The listing builds one solid part. Answer for the finished solid, in the listing's coordinates (mm). A direction names the side the tool comes from. Round coordinates to 2 decimals unless told otherwise and drop trailing zeros. Write each loop counter-clockwise with the first axis right and the second up, starting at its lowest first coordinate (ties: lowest second). Pieces come first, ordered by that corner, then holes.
from build123d import *

# Parameters (mm, degrees)
SKETCH1_W               = 10
SKETCH1_H               = 10
BOSS_EXTRUDE1_DEPTH     = 5
SKETCH4_R               = 3
CUT_EXTRUDE1_DEPTH      = 4
SKETCH5_R               = 4.05
BOSS_EXTRUDE2_DEPTH     = 30
CUT_EXTRUDE2_DEPTH      = 106.032848815
CUT_EXTRUDE2_DEPTH_BACK = 106.032848815
SKETCH6_W               = 26.365617629
SKETCH6_H               = 20
SKETCH8_W               = 10
SKETCH8_H               = 8.643528748
BOSS_EXTRUDE3_DEPTH     = 40
SKETCH9_R               = 2.5
BOSS_EXTRUDE4_DEPTH     = 10
CUT_EXTRUDE3_DEPTH      = 99.974452188
CUT_EXTRUDE3_DEPTH_BACK = 99.974452188
CUT_EXTRUDE5_DEPTH      = 99.974452188
CUT_EXTRUDE5_DEPTH_BACK = 99.974452188
SKETCH13_W              = 27.262735852
SKETCH13_H              = 14.70463532
SKETCH14_W              = 24
SKETCH14_H              = 18
BOSS_EXTRUDE5_DEPTH     = 10
SKETCH15_R              = 2.246907778
BOSS_EXTRUDE6_DEPTH     = 9
SKETCH16_W              = 26.867537366
SKETCH16_H              = 22.487326792
CUT_EXTRUDE6_DEPTH      = 5.25


with BuildPart() as part:
    # Sketch1 → Boss-Extrude1 (new, symmetric)
    with BuildSketch(Plane(origin=(0, 0, 0), x_dir=(0, 0, -1), z_dir=(1, 0, 0))):
        with BuildLine():
            Line((-40, -40), (-40, -50))
            Line((-40, -50), (-3.5, -50))
            ThreePointArc((-3.5, -50), (0, -46.5), (3.5, -50))
            Line((3.5, -50), (40, -50))
            Line((40, -50), (40, -40))
            Line((40, -40), (40, 50))
            Line((40, 50), (-40, 50))
            Line((-40, 50), (-40, -40))
        make_face()
        with Locations((-45, -45)):
            Rectangle(SKETCH1_W, SKETCH1_H)
        with Locations((45, -45)):
            Rectangle(SKETCH1_W, SKETCH1_H)
    extrude(amount=BOSS_EXTRUDE1_DEPTH, both=True)

    # Sketch4 → Cut-Extrude1 (cut)
    with BuildSketch(Plane(origin=(0, -40, 0), x_dir=(1, 0, 0), z_dir=(0, 1, 0))):
        with Locations(Location((0, -45, 0), (0, 0, 270))):
            Circle(SKETCH4_R)
    cut_extrude1 = extrude(amount=-CUT_EXTRUDE1_DEPTH, mode=Mode.SUBTRACT)

    # Mirror1: Cut-Extrude1 across plane
    add(cut_extrude1.mirror(Plane.XY), mode=Mode.SUBTRACT)

    # Sketch5 → Boss-Extrude2 (add, symmetric)
    with BuildSketch(Plane(origin=(0, 0, 0), x_dir=(1, 0, 0), z_dir=(0, 1, 0))):
        with BuildLine():
            Line((5, 15.751709746), (5, -15.751709746))
            Line((5, -15.751709746), (10, -15.751709746))
            Line((10, -15.751709746), (10, -8))
            Line((10, -8), (14.05, -8))
            ThreePointArc((14.05, -8), (17.885745365, -7.020474165), (20.782187809, -4.321764374))
            Line((20.782187809, -4.321764374), (20.782187809, 4.321764374))
            ThreePointArc((20.782187809, 4.321764374), (17.885745365, 7.020474165), (14.05, 8))
            Line((14.05, 8), (10, 8))
            Line((10, 8), (10, 15.751709746))
            Line((10, 15.751709746), (5, 15.751709746))
        make_face()
        with Locations(Location((14.05, 0, 0), (0, 0, 270))):
            Circle(SKETCH5_R, mode=Mode.SUBTRACT)
    extrude(amount=BOSS_EXTRUDE2_DEPTH, both=True)

    # Sketch6 → Cut-Extrude2 (cut, two sides: drawn at the far end of the back side and taken through both)
    with BuildSketch(Plane.XY.offset(40).offset(-CUT_EXTRUDE2_DEPTH_BACK)):
        with Locations((18.182808814, 0)):
            Rectangle(SKETCH6_W, SKETCH6_H)
    extrude(amount=CUT_EXTRUDE2_DEPTH + CUT_EXTRUDE2_DEPTH_BACK, mode=Mode.SUBTRACT)

    # Sketch8 → Boss-Extrude3 (add)
    with BuildSketch(Plane.XZ.offset(-10)):
        with Locations((25.782187809, 0)):
            Rectangle(SKETCH8_W, SKETCH8_H)
    extrude(amount=-BOSS_EXTRUDE3_DEPTH)

    # Sketch9 → Boss-Extrude4 (add)
    with BuildSketch(Plane.XY.offset(4.321764374)):
        with BuildLine():
            Line((30.782187809, 10), (54.782187809, 50))
            ThreePointArc((54.782187809, 50), (42.782187809, 62), (30.782187809, 50))
            Line((30.782187809, 50), (30.782187809, 10))
        make_face()
        with Locations((42.782187809, 57.067437711)):
            Circle(SKETCH9_R, mode=Mode.SUBTRACT)
    extrude(amount=-BOSS_EXTRUDE4_DEPTH)

    # Sketch10 → Cut-Extrude3 (cut, two sides: drawn at the far end of the back side and taken through both)
    with BuildSketch(Plane.XY.offset(4.321764374).offset(-CUT_EXTRUDE3_DEPTH_BACK)):
        Polygon((30.782187809, 50), (20.782187809, 30), (20.782187809, 50), align=None)
    extrude(amount=CUT_EXTRUDE3_DEPTH + CUT_EXTRUDE3_DEPTH_BACK, mode=Mode.SUBTRACT)

    # Sketch13 → Cut-Extrude5 (cut, two sides: drawn at the far end of the back side and taken through both)
    with BuildSketch(Plane.XY.offset(4.321764374).offset(-CUT_EXTRUDE5_DEPTH_BACK)):
        with Locations((44.413555735, 57.35231766)):
            Rectangle(SKETCH13_W, SKETCH13_H)
    extrude(amount=CUT_EXTRUDE5_DEPTH + CUT_EXTRUDE5_DEPTH_BACK, mode=Mode.SUBTRACT)

    # Sketch14 → Boss-Extrude5 (add)
    with BuildSketch(Plane(origin=(0, 50, 0), x_dir=(1, 0, 0), z_dir=(0, 1, 0))):
        with Locations((42.782187809, 0.678235626)):
            Rectangle(SKETCH14_W, SKETCH14_H)
    extrude(amount=-BOSS_EXTRUDE5_DEPTH)

    # Sketch15 → Boss-Extrude6 (add, symmetric)
    with BuildSketch(Plane.XY.offset(-0.678235626)):
        with BuildLine():
            Line((30.782187809, 50), (54.782187809, 50))
            Line((54.782187809, 50), (54.782187809, 61.15))
            ThreePointArc((54.782187809, 61.15), (42.783764567, 70.463225851), (30.782187809, 61.15406416))
            Line((30.782187809, 61.15406416), (30.782187809, 50))
        make_face()
        with Locations((42.782187809, 67.246907778)):
            Circle(SKETCH15_R, mode=Mode.SUBTRACT)
    extrude(amount=BOSS_EXTRUDE6_DEPTH, both=True)

    # Sketch16 → Cut-Extrude6 (cut, symmetric)
    with BuildSketch(Plane.XY.offset(-0.678235626)):
        with Locations((44.215956492, 61.243663396)):
            Rectangle(SKETCH16_W, SKETCH16_H)
    extrude(amount=CUT_EXTRUDE6_DEPTH, both=True, mode=Mode.SUBTRACT)


solid = part.part
1. Straight lines are drawn through the part: line 1 along Z through (x, y) = (45, 58.5); line 2 along Z through (x, y) = (14.05, 24); line 3 along X through (y, z) = (36, -19). For each, find the intervals that lie inside material, in ascending order.
Geometry says:
line 1: z = -9.68 to -5.93, 4.57 to 8.32
line 2: z = -8 to -4.05, 4.05 to 8
line 3: x = -5 to 5
2. A tool of negligible diameter and unlimited length cuts with its end or side. For faces 1 (the face through (12, 20, 8)), 2 (the face through (9, -10, 0)), 3 (the face through (12, -20, -8)), 4 (the face through (0, -42, 42)), from which of +Z, -Z, +X, -X, +Y, -Y can it reach the whole face along a straight path? Write none if from no direction.
Geometry says:
face 1: +Z, +X, +Y, -Y
face 2: +Z, -Z, +X
face 3: -Z, +X, +Y, -Y
face 4: +Y
3. Section A-A on z = 0 is taken. Determine the outline of the cut face in (x, y).
Geometry says:
outline: (-5, -46.5) - (5, -46.5) - (5, -30) - (10, -30) - (10, -10) - (5, -10) - (5, 10) - (10, 10) - (10, 30) - (5, 30) - (5, 50) - (-5, 50) - close; (18.1, -30) - (20.78, -30) - (20.78, -10) - (18.1, -10) - close; (18.1, 10) - (30.78, 10) - (48.78, 40) - (54.78, 40) - (54.78, 50) - (30.78, 50) - (20.78, 30) - (18.1, 30) - close
4. For a pull along Z with two mould halves and no side action, classify faces 5 (the face through (43, 50, -1)), 6 (the face through (43, 55, -9.678)), 7 (the face through (17.837, -19.86, 7.047)) as released by +Z, released by -Z, zero draft, split by the parting line, or undercut.
Geometry says:
face 5: undercut
face 6: released by -Z
face 7: released by +Z
5. Given pin 1 (8.5 mm diameter, centred on y = -18, z = -11, fed in from +X); pin 2 (5 mm diameter, centred on x = 27, y = 28, fed in from -Z); pin 3 (3.5 mm diameter, centred on x = 0, z = -45, fed in from +Y), each flat-ended and moving along its own axis, determine where each tip first touches the part or whether it passes through.
Geometry says:
pin 1: stops at x = 18.34
pin 2: stops at z = -4.32
pin 3: stops at y = -44
6. Section C-C on y = -25.5 is taken. Determine the outline of the cut face in (x, z), plus the area to 3 significant figures.
Geometry says:
outline: (-5, -40) - (5, -40) - (5, -15.75) - (10, -15.75) - (10, -8) - (14.05, -8) arc R8 ccw to (20.78, -4.32) - (20.78, 4.32) arc R8 ccw to (14.05, 8) - (10, 8) - (10, 15.75) - (5, 15.75) - (5, 40) - (-5, 40) - close; hole circle Ø8.1 at (14.05, 0)
area: 1,060 mm2
7. Section D-D on z = 45 is taken. Determine the outline of the cut face in (x, y), plus the area to 3 significant figures.
Geometry says:
outline: (-5, -50) - (5, -50) - (5, -40) - (3, -40) - (3, -44) - (-3, -44) - (-3, -40) - (-5, -40) - close
area: 76.0 mm2
8. Section B-B on y = 55.5 is taken. Determine the outline of the cut face in (x, z).
Geometry says:
outline: (30.78, -9.68) - (54.78, -9.68) - (54.78, -5.93) - (30.78, -5.93) - close; (30.78, 4.57) - (54.78, 4.57) - (54.78, 8.32) - (30.78, 8.32) - close
